```python
from build123d import *

# Parameters (mm, degrees)
SKETCH2_R           = 14.2875
SKETCH2_R_2         = 3.556
SKETCH2_R_3         = 3.175
BOSS_EXTRUDE1_DEPTH = 3.175


with BuildPart() as part:
    # Sketch2 → Boss-Extrude1 (new body)
    with BuildSketch(Plane(origin=(0, 0, 0), x_dir=(0, 0, -1), z_dir=(1, 0, 0))):
        with BuildLine():
            Line((-165.1, 19.05), (-65.425970741, 19.05))
            ThreePointArc((-65.425970741, 19.05), (-60.058718817, 17.860108895), (-55.697206313, 14.513402643))
            Line((-55.697206313, 14.513402643), (10.854621695, -64.799977479))
            ThreePointArc((10.854621695, -64.799977479), (17.220460091, -68.883236769), (24.778864428, -68.623566193))
            Line((24.778864428, -68.623566193), (101.178891774, -41.883356934))
            ThreePointArc((101.178891774, -41.883356934), (109.926930654, -35.593169628), (113.863183314, -25.563186798))
            Line((113.863183314, -25.563186798), (117.509534259, 16.114795214))
            ThreePointArc((117.509534259, 16.114795214), (115.335280515, 26.750250711), (107.704738864, 34.471333996))
            Line((107.704738864, 34.471333996), (35.042428799, 74.391177223))
            ThreePointArc((35.042428799, 74.391177223), (32.634742589, 76.723403199), (31.75, 79.956584517))
            Line((31.75, 79.956584517), (31.75, 123.825))
            ThreePointArc((31.75, 123.825), (29.890128061, 128.315128061), (25.4, 130.175))
            Line((25.4, 130.175), (-32.251185784, 130.175))
            ThreePointArc((-32.251185784, 130.175), (-36.116820858, 128.862793711), (-38.384814781, 125.468500936))
            Line((-38.384814781, 125.468500936), (-45.22073508, 99.956499064))
            ThreePointArc((-45.22073508, 99.956499064), (-47.488729003, 96.562206289), (-51.354364077, 95.25))
            Line((-51.354364077, 95.25), (-66.704490653, 95.25))
            ThreePointArc((-66.704490653, 95.25), (-67.533331973, 95.19567487), (-68.347991589, 95.033628997))
            Line((-68.347991589, 95.033628997), (-87.368500936, 89.937098878))
            ThreePointArc((-87.368500936, 89.937098878), (-90.762793711, 87.669104955), (-92.075, 83.803469881))
            Line((-92.075, 83.803469881), (-92.075, 50.8))
            ThreePointArc((-92.075, 50.8), (-93.934871939, 46.309871939), (-98.425, 44.45))
            Line((-98.425, 44.45), (-165.1, 44.45))
            ThreePointArc((-165.1, 44.45), (-167.34506403, 43.52006403), (-168.275, 41.275))
            Line((-168.275, 41.275), (-168.275, 22.225))
            ThreePointArc((-168.275, 22.225), (-167.34506403, 19.97993597), (-165.1, 19.05))
        make_face()
        Circle(SKETCH2_R, mode=Mode.SUBTRACT)
        with Locations((-53.975, 31.75)):
            Circle(SKETCH2_R_2, mode=Mode.SUBTRACT)
        with Locations((-79.375, 31.75)):
            Circle(SKETCH2_R_2, mode=Mode.SUBTRACT)
        with Locations((-104.775, 31.75)):
            Circle(SKETCH2_R_2, mode=Mode.SUBTRACT)
        with Locations((-130.175, 31.75)):
            Circle(SKETCH2_R_2, mode=Mode.SUBTRACT)
        with Locations((-155.575, 31.75)):
            Circle(SKETCH2_R_2, mode=Mode.SUBTRACT)
        with Locations((88.260023092, 2.022732411)):
            Circle(SKETCH2_R, mode=Mode.SUBTRACT)
        with Locations((-79.375, 57.15)):
            Circle(SKETCH2_R_2, mode=Mode.SUBTRACT)
        with Locations((-79.375, 82.55)):
            Circle(SKETCH2_R_2, mode=Mode.SUBTRACT)
        with Locations((21.222889041, -56.412747143)):
            Circle(SKETCH2_R_3, mode=Mode.SUBTRACT)
        with BuildLine():
            Line((94.576884308, 26.061982823), (94.799197401, 26.672783027))
            ThreePointArc((94.799197401, 26.672783027), (97.72919278, 28.03906231), (99.095472064, 25.109066932))
            Line((99.095472064, 25.109066932), (98.87315897, 24.498266728))
            ThreePointArc((98.87315897, 24.498266728), (95.943163592, 23.131987445), (94.576884308, 26.061982823))
        make_face(mode=Mode.SUBTRACT)
        with BuildLine():
            Line((66.519823852, -13.57854466), (65.937070193, -14.410803137))
            ThreePointArc((65.937070193, -14.410803137), (65.558381242, -16.118958605), (66.498456032, -17.594580444))
            ThreePointArc((66.498456032, -17.594580444), (78.790853404, -23.993597488), (92.320584973, -26.993066764))
            ThreePointArc((92.320584973, -26.993066764), (93.989235477, -26.466943281), (94.797124081, -24.915003712))
            Line((94.797124081, -24.915003712), (94.885674315, -23.902869899))
            ThreePointArc((94.885674315, -23.902869899), (94.359550833, -22.234219395), (92.807611263, -21.426330791))
            ThreePointArc((92.807611263, -21.426330791), (80.702061965, -18.742595123), (69.703601159, -13.01715882))
            ThreePointArc((69.703601159, -13.01715882), (67.995445691, -12.63846987), (66.519823852, -13.57854466))
        make_face(mode=Mode.SUBTRACT)
        with BuildLine():
            Line((-22.225, 117.475), (-22.225, 104.775))
            ThreePointArc((-22.225, 104.775), (-25.4, 101.6), (-28.575, 104.775))
            Line((-28.575, 104.775), (-28.575, 117.475))
            ThreePointArc((-28.575, 117.475), (-25.4, 120.65), (-22.225, 117.475))
        make_face(mode=Mode.SUBTRACT)
        with BuildLine():
            Line((15.875, 117.475), (15.875, 104.775))
            ThreePointArc((15.875, 104.775), (12.7, 101.6), (9.525, 104.775))
            Line((9.525, 104.775), (9.525, 117.475))
            ThreePointArc((9.525, 117.475), (12.7, 120.65), (15.875, 117.475))
        make_face(mode=Mode.SUBTRACT)
    extrude(amount=BOSS_EXTRUDE1_DEPTH)


solid = part.part
```
Model file for the job. Use its own axes, mm. A direction names the side the tool comes from. Coordinates: 2 decimals unless noted, no trailing zeros. Order: outer loops, then holes, each group sorted by start corner. A loop starts at its lowest first (then second) coordinate and runs counter-clockwise, first axis right, second up. Notation, with made-up numbers: (21, 60) - (44, 60) arc R30 cw to (44, 91) - close; hole circle Ø3 at (-7, -9). An arc over 180 degrees is marked (long way). Return JSON: item names as keys, results as strings. Group by question number.
1) Probe line 1 (Z direction, x = 0.75, y = 115) (3 decimals); line 2 (Y direction, x = 2.05, z = 130); line 3 (Y direction, x = 1.05, z = -6) (3 decimals). List the from-to ranges inside material, lowest first. Write a range as from..to.
2) Saw through at A-A, the plane z = 25.4. Write the cut outline in (x, y) (3 decimals).
3) Saw through at C-C, the plane y = 57.15. Write the cut outline in (x, z) (3 decimals), plus the area to 3 significant figures.
4) Tool access for faces 1 (the flat face through (1.565, -24.588, 22.887)), 2 (the cylindrical face through (1.565, -18.802, -80.866)): list every direction of +Z, -Z, +X, -X, +Y, -Y with a clear straight run to the whole face (end or side of a thin tool).
5) Saw through at B-B, the plane z = 79. Write the cut outline in (x, y) (3 decimals).
6) Mould opens along Y. For faces 3 (the flat face through (1.57, -55.44, -62.44)), 4 (the cylindrical face through (1.57, 30.39, 126.89)), 5 (the cylindrical face through (1.565, 46.36, 93.886)), 6 (the flat face through (3.175, 32, -4)) say: released by +Y, released by -Y, zero draft, split by the parting line, or undercut.
7) Saw through at D-D, the plane x = 1.7. Count the separate pieces of the cut face and the enclosed holes in it, plus the area to 3 significant figures.
Values found:
{
 "1": {"line 1": "z = -31.75..-15.875, -9.525..22.225, 28.575..41.19", "line 2": "y = 19.05..28.2, 35.3..44.45", "line 3": "y = -59.014..-12.967, 12.967..130.175"},
 "2": {"outline": "(0, -21.593) - (3.175, -21.593) - (3.175, 101.6) - (0, 101.6) - close; (0, 120.65) - (3.175, 120.65) - (3.175, 130.175) - (0, 130.175) - close"},
 "3": {"outline": "(0, -66.425) - (3.175, -66.425) - (3.175, 75.819) - (0, 75.819) - close; (0, 82.931) - (3.175, 82.931) - (3.175, 92.075) - (0, 92.075) - close", "area": "481 mm²"},
 "4": {"face 1": "+Z, +X, -X, -Y", "face 2": "+X, -X"},
 "5": {"outline": "(0, 19.05) - (3.175, 19.05) - (3.175, 28.214) - (0, 28.214) - close; (0, 35.286) - (3.175, 35.286) - (3.175, 53.614) - (0, 53.614) - close; (0, 60.686) - (3.175, 60.686) - (3.175, 79.014) - (0, 79.014) - close; (0, 86.086) - (3.175, 86.086) - (3.175, 92.179) - (0, 92.179) - close"},
 "6": {"face 3": "released by -Y", "face 4": "undercut", "face 5": "released by +Y", "face 6": "zero draft"},
 "7": {"separate pieces": "1", "enclosed holes": "14", "area": "25,400 mm²"}
}
